Source: CAD feature listing. Evaluate the final solid. Frame: model axes, mm. Coordinates: 2 decimals unless noted, no trailing zeros. Loops run counter-clockwise (first coordinate to the right, second up) from the corner with the lowest first, then second, coordinate; pieces in that order, holes last.
Item 1: Section query A-A, the plane z = -25.5. Return the cut outline in (x, y), then the cut area to 3 significant figures.
Item 2: Section query B-B, the plane x = 68.5. Return the cut outline in (y, z).
Item 3: Line query: probe 1 along X at (y, z) = (1.35, -27); probe 2 along X at (y, z) = (2.35, -21.25); probe 3 along Z at (x, y) = (119, 2). Output: solid intervals per line, ascending.
Item 4: Pin query (flat end, axial travel): pin 1 Ø3 at (x, y) = (69.5, 3.5) entering from -Z. Return the tip coordinate at first contact, or that it passes through.
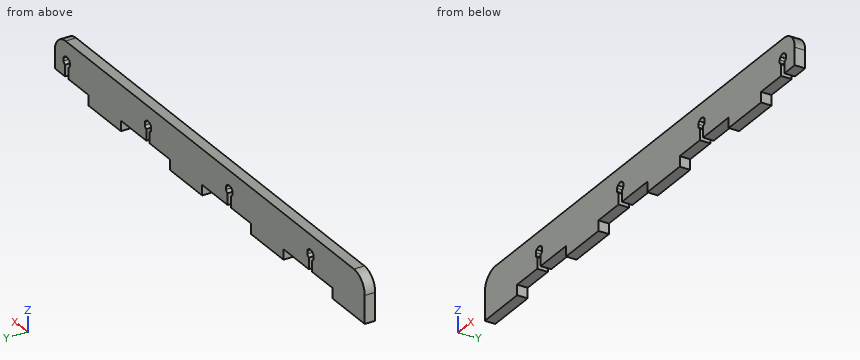
```python
from build123d import *

# Parameters (mm, degrees)
SALIENTE_EXTRUIR1_DEPTH = 6


with BuildPart() as part:
    # Croquis1 → Saliente-Extruir1 (new body)
    with BuildSketch(Plane(origin=(0, 0, 0), x_dir=(1, 0, 0), z_dir=(0, 1, 0))):
        with BuildLine():
            ThreePointArc((-95.152264236, 14.320303243), (-94.78653124, 15.320309075), (-93.861926606, 15.848398611))
            Line((-93.861926606, 15.848398611), (-93.861926606, 22.348623853))
            Line((-93.861926606, 22.348623853), (-112.411926606, 22.348623853))
            Line((-112.411926606, 22.348623853), (-112.411926606, 28.248623853))
            Line((-112.411926606, 28.248623853), (-142.311926606, 28.248623853))
            Line((-142.311926606, 28.248623853), (-142.311926606, 22.348623853))
            Line((-142.311926606, 22.348623853), (-142.311926606, 12.348623853))
            ThreePointArc((-142.311926606, 12.348623853), (-139.382994417, 5.277556041), (-132.311926606, 2.348623853))
            Line((-132.311926606, 2.348623853), (127.688073394, 2.348623853))
            Line((127.688073394, 2.348623853), (133.688073394, 2.348623853))
            ThreePointArc((133.688073394, 2.348623853), (140.759141206, 5.277556041), (143.688073394, 12.348623853))
            Line((143.688073394, 12.348623853), (143.688073394, 22.348623853))
            Line((143.688073394, 22.348623853), (137.688073394, 22.348623853))
            Line((137.688073394, 22.348623853), (134.238073394, 22.348623853))
            Line((134.238073394, 22.348623853), (134.238073394, 15.848398611))
            ThreePointArc((134.238073394, 15.848398611), (135.162678029, 15.320309075), (135.528411025, 14.320303243))
            Line((135.528411025, 14.320303243), (135.528411025, 12.770303243))
            ThreePointArc((135.528411025, 12.770303243), (135.339714195, 12.029119271), (134.819567568, 11.468398611))
            Line((134.819567568, 11.468398611), (134.650322636, 11.468398611))
            ThreePointArc((134.650322636, 11.468398611), (132.688073394, 10.655388626), (130.725824153, 11.468398611))
            Line((130.725824153, 11.468398611), (130.556579221, 11.468398611))
            ThreePointArc((130.556579221, 11.468398611), (130.036432594, 12.029119271), (129.847735764, 12.770303243))
            Line((129.847735764, 12.770303243), (129.847735764, 14.320303243))
            ThreePointArc((129.847735764, 14.320303243), (130.21346876, 15.320309075), (131.138073394, 15.848398611))
            Line((131.138073394, 15.848398611), (131.138073394, 22.348623853))
            Line((131.138073394, 22.348623853), (112.588073394, 22.348623853))
            Line((112.588073394, 22.348623853), (112.588073394, 28.248623853))
            Line((112.588073394, 28.248623853), (82.688073394, 28.248623853))
            Line((82.688073394, 28.248623853), (82.688073394, 22.348623853))
            Line((82.688073394, 22.348623853), (59.238073394, 22.348623853))
            Line((59.238073394, 22.348623853), (59.238073394, 15.848398611))
            ThreePointArc((59.238073394, 15.848398611), (60.162678029, 15.320309075), (60.528411025, 14.320303243))
            Line((60.528411025, 14.320303243), (60.528411025, 12.770303243))
            ThreePointArc((60.528411025, 12.770303243), (60.339714195, 12.029119271), (59.819567568, 11.468398611))
            Line((59.819567568, 11.468398611), (59.650322636, 11.468398611))
            ThreePointArc((59.650322636, 11.468398611), (57.688073394, 10.655388626), (55.725824153, 11.468398611))
            Line((55.725824153, 11.468398611), (55.556579221, 11.468398611))
            ThreePointArc((55.556579221, 11.468398611), (55.036432594, 12.029119271), (54.847735764, 12.770303243))
            Line((54.847735764, 12.770303243), (54.847735764, 14.320303243))
            ThreePointArc((54.847735764, 14.320303243), (55.21346876, 15.320309075), (56.138073394, 15.848398611))
            Line((56.138073394, 15.848398611), (56.138073394, 22.348623853))
            Line((56.138073394, 22.348623853), (37.588073394, 22.348623853))
            Line((37.588073394, 22.348623853), (37.588073394, 28.248623853))
            Line((37.588073394, 28.248623853), (7.688073394, 28.248623853))
            Line((7.688073394, 28.248623853), (7.688073394, 22.348623853))
            Line((7.688073394, 22.348623853), (-15.761926606, 22.348623853))
            Line((-15.761926606, 22.348623853), (-15.761926606, 15.848398611))
            ThreePointArc((-15.761926606, 15.848398611), (-14.837321971, 15.320309075), (-14.471588975, 14.320303243))
            Line((-14.471588975, 14.320303243), (-14.471588975, 12.770303243))
            ThreePointArc((-14.471588975, 12.770303243), (-14.660285805, 12.029119271), (-15.180432432, 11.468398611))
            Line((-15.180432432, 11.468398611), (-15.349677364, 11.468398611))
            ThreePointArc((-15.349677364, 11.468398611), (-17.311926606, 10.655388626), (-19.274175847, 11.468398611))
            Line((-19.274175847, 11.468398611), (-19.443420779, 11.468398611))
            ThreePointArc((-19.443420779, 11.468398611), (-19.963567406, 12.029119271), (-20.152264236, 12.770303243))
            Line((-20.152264236, 12.770303243), (-20.152264236, 14.320303243))
            ThreePointArc((-20.152264236, 14.320303243), (-19.78653124, 15.320309075), (-18.861926606, 15.848398611))
            Line((-18.861926606, 15.848398611), (-18.861926606, 22.348623853))
            Line((-18.861926606, 22.348623853), (-37.411926606, 22.348623853))
            Line((-37.411926606, 22.348623853), (-37.411926606, 28.248623853))
            Line((-37.411926606, 28.248623853), (-67.311926606, 28.248623853))
            Line((-67.311926606, 28.248623853), (-67.311926606, 22.348623853))
            Line((-67.311926606, 22.348623853), (-90.761926606, 22.348623853))
            Line((-90.761926606, 22.348623853), (-90.761926606, 15.848398611))
            ThreePointArc((-90.761926606, 15.848398611), (-89.837321971, 15.320309075), (-89.471588975, 14.320303243))
            Line((-89.471588975, 14.320303243), (-89.471588975, 12.770303243))
            ThreePointArc((-89.471588975, 12.770303243), (-89.660285805, 12.029119271), (-90.180432432, 11.468398611))
            Line((-90.180432432, 11.468398611), (-90.349677364, 11.468398611))
            ThreePointArc((-90.349677364, 11.468398611), (-92.311926606, 10.655388626), (-94.274175847, 11.468398611))
            Line((-94.274175847, 11.468398611), (-94.443420779, 11.468398611))
            ThreePointArc((-94.443420779, 11.468398611), (-94.963567406, 12.029119271), (-95.152264236, 12.770303243))
            Line((-95.152264236, 12.770303243), (-95.152264236, 14.320303243))
        make_face()
    extrude(amount=SALIENTE_EXTRUIR1_DEPTH)


solid = part.part
```
Verdict:
1. outline: (-142.31, 0) - (-112.41, 0) - (-112.41, 6) - (-142.31, 6) - close; (-67.31, 0) - (-37.41, 0) - (-37.41, 6) - (-67.31, 6) - close; (7.69, 0) - (37.59, 0) - (37.59, 6) - (7.69, 6) - close; (82.69, 0) - (112.59, 0) - (112.59, 6) - (82.69, 6) - close
1. area: 718 mm2
2. outline: (0, -22.35) - (6, -22.35) - (6, -2.35) - (0, -2.35) - close
3. probe 1: x = -142.31 to -112.41, -67.31 to -37.41, 7.69 to 37.59, 82.69 to 112.59
3. probe 2: x = -142.31 to -93.86, -90.76 to -18.86, -15.76 to 56.14, 59.24 to 131.14, 134.24 to 143.69
3. probe 3: z = -22.35 to -2.35
4. pin 1: stops at z = -22.35
